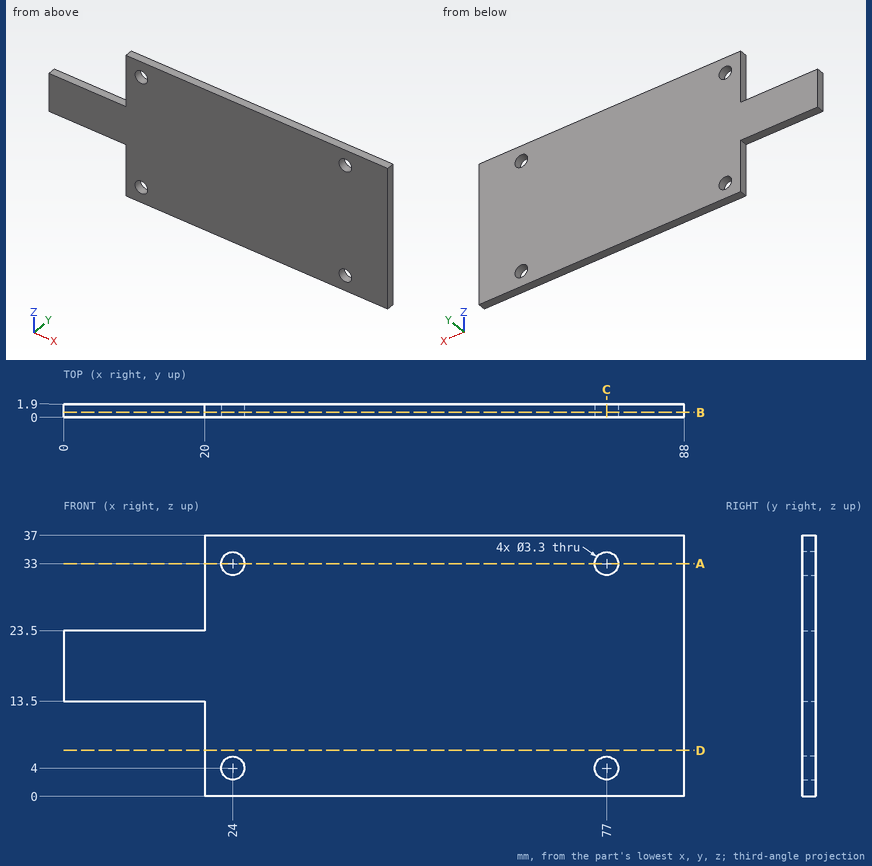
Drawing for the job (mm, zero at the part's lowest x, y, z). Give positions to 0.01 mm unless a question says otherwise; leave off trailing zeros. Write each loop counter-clockwise with the first axis right and the second up, starting at its lowest first coordinate (ties: lowest second). Pieces come first, ordered by that corner, then holes. Notation, with made-up numbers: M -4,20.5 L 32,20.5 A7 ccw 32,27.5 Z; hole C 17,64 d8. An arc over 180 degrees is marked long. Return JSON: item names as keys, results as strings. Group by question number.
(1) Drill centre lines: L1, parallel to Z at x = 24, y = 1.15; L2, parallel to X at y = 1, z = 4; L3, parallel to X at y = 0.9, z = 34. Where is each one in solid material? Low to high. Write a range as [from, to].
(2) Band-saw the part on A-A (z = 33). Give the cut face in (x, y), and give its area (3 significant figures).
(3) Band-saw the part on D-D (z = 6.5). Give the cut face in (x, y), and give its area (3 significant figures).
(4) Band-saw the part on B-B (y = 0.7). Give the cut face in (x, z).
(5) Flat gauge pins, fed straight in: pin 1 Ø2 at (x, z) = (20.5, 12) entering from -Y; pin 2 Ø3 at (x, z) = (77, 33) entering from -Y; pin 3 Ø0.6 at (x, y) = (11.5, 1) entering from -Z. Where does each tip first touch, or does it go through?
(6) Band-saw the part on C-C (x = 77). Give the cut face in (y, z).
Entries:
{
 "1": {"L1": "z = [0, 2.35], [5.65, 31.35], [34.65, 37]", "L2": "x = [20, 22.35], [25.65, 75.35], [78.65, 88]", "L3": "x = [20, 22.69], [25.31, 75.69], [78.31, 88]"},
 "2": {"outline": "M 20,0 L 22.35,0 L 22.35,1.9 L 20,1.9 Z; M 25.65,0 L 75.35,0 L 75.35,1.9 L 25.65,1.9 Z; M 78.65,0 L 88,0 L 88,1.9 L 78.65,1.9 Z", "area": "117 mm^2"},
 "3": {"outline": "M 20,0 L 88,0 L 88,1.9 L 20,1.9 Z", "area": "129 mm^2"},
 "4": {"outline": "M 0,13.5 L 20,13.5 L 20,0 L 88,0 L 88,37 L 20,37 L 20,23.5 L 0,23.5 Z; hole C 24,4 d3.3; hole C 24,33 d3.3; hole C 77,4 d3.3; hole C 77,33 d3.3"},
 "5": {"pin 1": "stops at y = 0", "pin 2": "passes through", "pin 3": "stops at z = 13.5"},
 "6": {"outline": "M 0,0 L 1.9,0 L 1.9,2.35 L 0,2.35 Z; M 0,5.65 L 1.9,5.65 L 1.9,31.35 L 0,31.35 Z; M 0,34.65 L 1.9,34.65 L 1.9,37 L 0,37 Z"}
}
